Build history of the part. All positions in model axes, mm. Face numbers are marked on the shaded views. A direction names the side the tool comes from. Round coordinates to 2 decimals unless told otherwise and drop trailing zeros. Loops run counter-clockwise (first coordinate to the right, second up) from the corner with the lowest first, then second, coordinate; pieces in that order, holes last. Notation, with made-up numbers: M 54.25,69 L 85.25,69 A25 ccw 85.25,100 Z; hole C 60,-39.5 d1. An arc over 180 degrees is marked long. Write each question's results on one line, items separated by ' | '. Start each with the question number.
```python
from build123d import *

# Parameters (mm, degrees)
F2_W      = 32
F2_H      = 24
F3_DEPTH  = 2
F0_W      = 24
F0_H      = 24
F4_DEPTH  = 3
F1_R      = 10
F5_DEPTH  = 3
F6_W      = 2
F6_H      = 20
F7_DEPTH  = 2
F8_R      = 2
F9_R      = 1
F10_W     = 10
F10_H     = 3
F11_DEPTH = 1
F12_DEPTH = 2
F13_W     = 4
F13_H     = 1.5
F14_DEPTH = 2
F15_SIZE  = 1
F16_R     = 0.5


with BuildPart() as f3:
    # F2 (on Top) → F3 (new body)
    with BuildSketch(Plane.XY):
        Rectangle(F2_W, F2_H)
    extrude(amount=F3_DEPTH)

    # F0 (on Top) → F4 (join)
    with BuildSketch(Plane.XY):
        Rectangle(F0_W, F0_H)
    extrude(amount=-F4_DEPTH)

    # F1 (on Top) → F5 (cut)
    with BuildSketch(Plane.XY):
        Circle(F1_R)
    extrude(amount=-F5_DEPTH, mode=Mode.SUBTRACT)

    # F6 (on Top) → F7 (cut)
    with BuildSketch(Plane.XY):
        with Locations((-13, 0)):
            Rectangle(F6_W, F6_H)
        with Locations((13, 0)):
            Rectangle(F6_W, F6_H)
    extrude(amount=F7_DEPTH, mode=Mode.SUBTRACT)

    # F8
    f8_edges = [f3.edges().sort_by_distance(p)[0] for p in [
        (16, -12, 1),
        (16, 12, 1),
        (-16, -12, 1),
        (-16, 12, 1),
    ]]
    fillet(f8_edges, radius=F8_R)

    # F9
    f9_edges = [f3.edges().sort_by_distance(p)[0] for p in [
        (-14, 10, 1),
        (14, 10, 1),
        (-14, -10, 1),
        (14, -10, 1),
    ]]
    fillet(f9_edges, radius=F9_R)

    # F10 (on Top) → F11 (cut)
    with BuildSketch(Plane.XY):
        with Locations((0, -10.5)):
            Rectangle(F10_W, F10_H)
    extrude(amount=-F11_DEPTH, mode=Mode.SUBTRACT)

    # F10 (on Top) → F12 (cut)
    with BuildSketch(Plane.XY):
        with Locations((0, -10.5)):
            Rectangle(F10_W, F10_H)
    extrude(amount=F12_DEPTH, mode=Mode.SUBTRACT)

    # F13 (on Top) → F14 (join)
    with BuildSketch(Plane.XY):
        with Locations((-7, -12.75)):
            Rectangle(F13_W, F13_H)
        with Locations((-7, 12.75)):
            Rectangle(F13_W, F13_H)
        with Locations((7, -12.75)):
            Rectangle(F13_W, F13_H)
        with Locations((7, 12.75)):
            Rectangle(F13_W, F13_H)
    extrude(amount=-F14_DEPTH)

    # F15
    f15_edges = [f3.edges().sort_by_distance(p)[0] for p in [
        (-7, -13.5, -2),
        (7, -13.5, -2),
        (7, 13.5, -2),
        (-7, 13.5, -2),
    ]]
    chamfer(f15_edges, length=F15_SIZE)

    # F16
    f16_edges = [f3.edges().sort_by_distance(p)[0] for p in [
        (0, -12, -3),
        (0, 12, -3),
    ]]
    fillet(f16_edges, radius=F16_R)


solid = f3.part
```
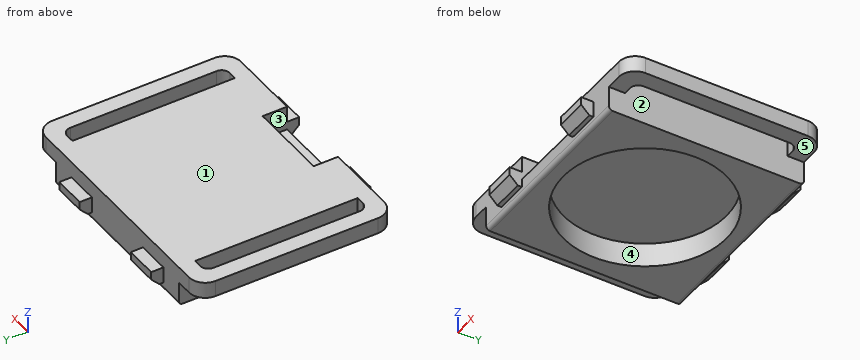
Item 1: Drill centre lines: line 1 along X through (y, z) = (3.5, 0.75); line 2 along X through (y, z) = (0, -0.75). Where is each one in solid material? Low to high. Write a range as [from, to].
Item 2: Mould opens along Y. For the marked faces 1 and 2 say: released by +Y, released by -Y, zero draft, split by the parting line, or undercut.
Item 3: Drop flat-ended pins along their axis: pin 1 (5 mm diameter, centred on x = -1, y = 4.5, fed in from -Z); pin 2 (1.3 mm diameter, centred on x = -1, z = -1, fed in from -Y); pin 3 (1.6 mm diameter, centred on y = -13, z = -0.5, fed in from +X). Give the stop position or say it passes through.
Item 4: Saw through at C-C, the plane x = -8. Give the cut face in (y, z), then the cut area to 3 significant figures.
Item 5: Tool access for the marked faces 3, 4 and 5: list every direction of +Z, -Z, +X, -X, +Y, -Y with a clear straight run to the whole face (end or side of a thin tool).
Item 6: Saw through at D-D, the plane y = -5.5. Give the cut face in (x, z).
Item 7: Saw through at A-A, the plane y = 0. Give the cut face in (x, z), then the cut area to 3 significant figures.
Item 8: Saw through at B-B, the plane x = 0. Give the cut face in (y, z).
Working result:
1) line 1: x = [-16, -14], [-12, 12], [14, 16] | line 2: x = [-12, -10], [10, 12]
2) face 1: zero draft | face 2: undercut
3) pin 1: stops at z = 0 | pin 2: stops at y = -12 | pin 3: stops at x = 9
4) outline: M -13.5,-1 L -12.5,-2 L -12,-2 L -12,-2.5 A0.5 ccw -11.5,-3 L -6,-3 L -6,0 L 6,0 L 6,-3 L 11.5,-3 A0.5 ccw 12,-2.5 L 12,-2 L 12.5,-2 L 13.5,-1 L 13.5,0 L 12,0 L 12,2 L -12,2 L -12,0 L -13.5,0 Z | area: 88.9 mm²
5) face 3: +Z, -Y | face 4: -Z | face 5: -Z, +X, +Y, -Y
6) outline: M -16,0 L -14,0 L -14,2 L -16,2 Z; M -12,-3 L -8.35,-3 L -8.35,0 L 8.35,0 L 8.35,-3 L 12,-3 L 12,2 L -12,2 Z; M 14,0 L 16,0 L 16,2 L 14,2 Z
7) outline: M -16,0 L -14,0 L -14,2 L -16,2 Z; M -12,-3 L -10,-3 L -10,0 L 10,0 L 10,-3 L 12,-3 L 12,2 L -12,2 Z; M 14,0 L 16,0 L 16,2 L 14,2 Z | area: 68.0 mm²
8) outline: M -12,-2.5 A0.5 ccw -11.5,-3 L -10,-3 L -10,-1 L -12,-1 Z; M -9,0 L 10,0 L 10,-3 L 11.5,-3 A0.5 ccw 12,-2.5 L 12,2 L -9,2 Z
